Part model, mm, in its own coordinate system. A direction names the side the tool comes from. Round coordinates to 2 decimals unless told otherwise and drop trailing zeros. Write each loop counter-clockwise with the first axis right and the second up, starting at its lowest first coordinate (ties: lowest second). Pieces come first, ordered by that corner, then holes.
```python
from build123d import *

# Parameters (mm, degrees)
BOSS_EXTRUDE1_DEPTH = 24
SKETCH3_W           = 7
SKETCH3_H           = 75
CUT_EXTRUDE1_DEPTH  = 21
SKETCH4_W           = 81
SKETCH4_H           = 12
CUT_EXTRUDE2_DEPTH  = 7
SKETCH5_R           = 2
CUT_EXTRUDE3_DEPTH  = 3


with BuildPart() as part:
    # Sketch2 → Boss-Extrude1 (new body)
    with BuildSketch(Plane.XY):
        Polygon((0, 0), (0, -75), (118, -75), (118, 0), (102, 0), (102, 12), (21, 12), (21, 0), align=None)
    extrude(amount=-BOSS_EXTRUDE1_DEPTH)

    # Sketch3 → Cut-Extrude1 (cut)
    with BuildSketch(Plane.XY):
        with Locations((3.5, -37.5)):
            Rectangle(SKETCH3_W, SKETCH3_H)
        with Locations((114.5, -37.5)):
            Rectangle(SKETCH3_W, SKETCH3_H)
    extrude(amount=-CUT_EXTRUDE1_DEPTH, mode=Mode.SUBTRACT)

    # Sketch4 → Cut-Extrude2 (cut)
    with BuildSketch(Plane.XY):
        with Locations((61.5, 6)):
            Rectangle(SKETCH4_W, SKETCH4_H)
    cut_extrude2 = extrude(amount=-CUT_EXTRUDE2_DEPTH, mode=Mode.SUBTRACT)

    # Mirror1: Cut-Extrude2 across plane
    add(cut_extrude2.mirror(Plane.XY.offset(-12)), mode=Mode.SUBTRACT)

    # Sketch5 → Cut-Extrude3 (cut)
    with BuildSketch(Plane(origin=(0, 0, -24), x_dir=(-1, 0, 0), z_dir=(0, 0, -1))):
        with Locations((-114.75, -26.25)):
            Circle(SKETCH5_R)
        with Locations((-114.75, -48.75)):
            Circle(SKETCH5_R)
        with Locations(Location((-3.25, -48.75, 0), (0, 0, 180))):
            Circle(SKETCH5_R)
        with Locations(Location((-3.25, -26.25, 0), (0, 0, 180))):
            Circle(SKETCH5_R)
    extrude(amount=-CUT_EXTRUDE3_DEPTH, mode=Mode.SUBTRACT)


solid = part.part
```
Q1. Mould opens along X. For faces 5 (the cylindrical face through (116.337, -49.967, -22.521)), 6 (the flat face through (7, -38, -10)), 7 (the flat face through (102, 6, -12)), 8 (the flat face through (62, 12, -12)) say: +X half, -X half, draft (parallel to the pull), parting line (faces both ways), or undercut.
Values follow:
face 5: undercut
face 6: -X half
face 7: +X half
face 8: draft
Q2. Drop flat-ended pins along their axis: pin 1 (6.5 mm diameter, centred on x = 114.75, y = -48.75, fed in from +Z); pin 2 (6 mm diameter, centred on y = -43.5, z = -17, fed in from -X); pin 3 (5 mm diameter, centred on y = 9, z = -10, fed in from -X). Give the stop position or say it passes through.
Values follow:
pin 1: stops at z = -21
pin 2: stops at x = 7
pin 3: stops at x = 21
Q3. Which spindle directions (+Z, -Z, +X, -X, +Y, -Y) get a long thin tool onto all of the face, cutting with end or side? Do faces 1 (the flat face through (61, 6, -17)), 2 (the flat face through (111, -38, -10)), 3 (the flat face through (61, 6, -7)), 4 (the flat face through (3, -37, -21)). Say none if no direction does.
Values follow:
face 1: -Z, +X, -X, +Y
face 2: +Z, +X, +Y, -Y
face 3: +Z, +X, -X, +Y
face 4: +Z, -X, +Y, -Y
Q4. Wall check: L1, parallel to Y at x = 114.75, z = -21.8; L2, parallel to X at y = -71, z = -3.5; L3, parallel to Y at x = 56.5, z = -5.5. Give the ranges that are in metal, low to high.
Values follow:
L1: y = -75 to -50.75, -46.75 to -28.25, -24.25 to 0
L2: x = 7 to 111
L3: y = -75 to 0
Q5. Cut at D-D on y = -5. Write the cut outline in (x, z), plus the area to 3 significant figures.
Values follow:
outline: (0, -24) - (118, -24) - (118, -21) - (111, -21) - (111, 0) - (7, 0) - (7, -21) - (0, -21) - close
area: 2,540 mm2
Q6. Cut at A-A on x = 114.75. Write the cut outline in (y, z), plus the area to 3 significant figures.
Values follow:
outline: (-75, -24) - (-50.75, -24) - (-50.75, -21) - (-75, -21) - close; (-46.75, -24) - (-28.25, -24) - (-28.25, -21) - (-46.75, -21) - close; (-24.25, -24) - (0, -24) - (0, -21) - (-24.25, -21) - close
area: 201 mm2
Q7. Cut at B-B on y = -48.75. Write the cut outline in (x, z).
Values follow:
outline: (0, -24) - (1.25, -24) - (1.25, -21) - (0, -21) - close; (5.25, -24) - (112.75, -24) - (112.75, -21) - (111, -21) - (111, 0) - (7, 0) - (7, -21) - (5.25, -21) - close; (116.75, -24) - (118, -24) - (118, -21) - (116.75, -21) - close
Q8. Cut at C-C on x = 34. Write the cut outline in (y, z).
Values follow:
outline: (-75, -24) - (0, -24) - (0, -17) - (12, -17) - (12, -7) - (0, -7) - (0, 0) - (-75, 0) - close
